For this review, take the finished solid that the model builds, in its own axes (mm). Face numbers are marked on the shaded views. A direction names the side the tool comes from. Coordinates: 2 decimals unless noted, no trailing zeros. Order: outer loops, then holes, each group sorted by start corner. A loop starts at its lowest first (then second) coordinate and runs counter-clockwise, first axis right, second up. Notation, with made-up numbers: (30, -6.5) -> (80, -6.5) arc R18 ccw to (80, 9.5) -> close; hole circle Ø3 at (54, 37.5). An arc over 180 degrees is marked (long way). Write item = value, one per line. Start each with the question number.
1) Draft analysis for pull direction Z (two halves, no side actions). For the marked faces 6, 7 and 8, state which applies: +Z half, -Z half, draft (parallel to the pull), parting line (faces both ways), or undercut.
2) Consider section A-A on x = -27. Give the boundary of the cut face in (y, z).
3) Consider section B-B on y = 17. Give the boundary of the cut face in (x, z), and give its area (3 significant figures).
4) Machinability: for the marked faces 1, 2, 3, 4 and 5, which of the approach directions +Z, -Z, +X, -X, +Y, -Y give a long, thin tool a straight path to every point of the face, cutting with its end or side? Answer none if there is none.
5) Consider section C-C on z = -17. Give the boundary of the cut face in (x, y).
6) Insertion check: pin 1 Ø5 at (x, z) = (-29, -9) entering from +Y; pin 2 Ø3 at (y, z) = (13, -1) entering from -X; pin 3 Ø3 at (x, z) = (-17.5, 9.5) entering from +Y. Each pin has a flat end and moves straight along its axis. Give the tip position at first contact, or say it passes through.
7) Consider section D-D on y = 6. Give the boundary of the cut face in (x, z).
8) Wall thickness on probe 1 along Z at (x, y) = (26, 5); probe 2 along X at (y, z) = (3, 0); probe 3 along Y at (x, z) = (-28, 7): over which ranges is each line inside the solid? List them lowest first. Write a range as [from, to].
from build123d import *

# Parameters (mm, degrees)
SALIENTE_EXTRUIR1_DEPTH = 20
CORTAR_EXTRUIR2_REACH   = 62.415
CROQUIS2_W              = 15
CROQUIS2_H              = 10


with BuildPart() as part:
    # Croquis1 → Saliente-Extruir1 (new, symmetric)
    with BuildSketch(Plane.XY):
        Polygon((-35, 0), (35, 0), (35, 10), (25, 10), (10, 45), (-10, 45), (-25, 10), (-35, 10), align=None)
    extrude(amount=SALIENTE_EXTRUIR1_DEPTH, both=True)

    # Croquis2 → Cortar-Extruir2 (cut, up to next)
    with BuildSketch(Plane.XZ, mode=Mode.PRIVATE) as cortar_extruir2_sk1:
        with Locations((27.5, 0)):
            Rectangle(CROQUIS2_W, CROQUIS2_H)
    cortar_extruir2_tool1 = extrude(cortar_extruir2_sk1.sketch, amount=-CORTAR_EXTRUIR2_REACH, mode=Mode.PRIVATE) & part.part
    # Croquis2 → Cortar-Extruir2 (cut, up to next)
    with BuildSketch(Plane.XZ, mode=Mode.PRIVATE) as cortar_extruir2_sk2:
        with Locations((-27.5, 0)):
            Rectangle(CROQUIS2_W, CROQUIS2_H)
    cortar_extruir2_tool2 = extrude(cortar_extruir2_sk2.sketch, amount=-CORTAR_EXTRUIR2_REACH, mode=Mode.PRIVATE) & part.part
    add(cortar_extruir2_tool1.solids().sort_by_distance((27.5, 0, 0))[0], mode=Mode.SUBTRACT)
    add(cortar_extruir2_tool2.solids().sort_by_distance((-27.5, 0, 0))[0], mode=Mode.SUBTRACT)


solid = part.part
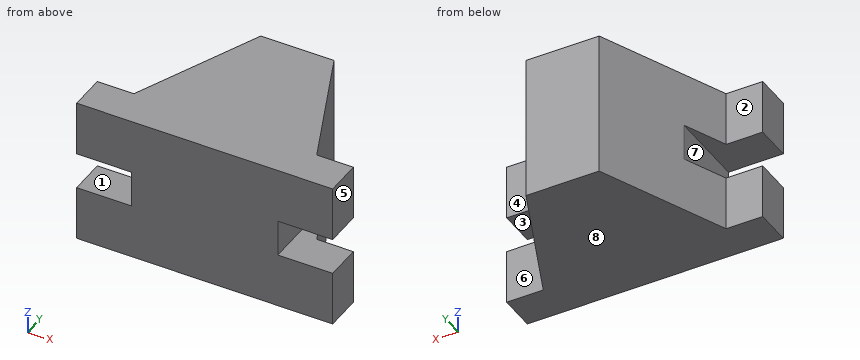
Answer sheet:
q1.face_6 = draft
q1.face_7 = undercut
q1.face_8 = -Z half
q2.outline = (0, -20) -> (10, -20) -> (10, -5) -> (0, -5) -> close; (0, 5) -> (10, 5) -> (10, 20) -> (0, 20) -> close
q3.outline = (-22, -20) -> (22, -20) -> (22, -5) -> (20, -5) -> (20, 5) -> (22, 5) -> (22, 20) -> (-22, 20) -> (-22, 5) -> (-20, 5) -> (-20, -5) -> (-22, -5) -> close
q3.area = 1,720 mm2
q4.face_1 = -X, +Y, -Y
q4.face_2 = +Z, -Z, -X, +Y
q4.face_3 = +X, +Y, -Y
q4.face_4 = +Z, -Z, +X, +Y
q4.face_5 = +Z, -Z, +X, +Y, -Y
q5.outline = (-35, 0) -> (35, 0) -> (35, 10) -> (25, 10) -> (10, 45) -> (-10, 45) -> (-25, 10) -> (-35, 10) -> close
q6.pin_1 = 10
q6.pin_2 = -20
q6.pin_3 = 31
q7.outline = (-35, -20) -> (35, -20) -> (35, -5) -> (20, -5) -> (20, 5) -> (35, 5) -> (35, 20) -> (-35, 20) -> (-35, 5) -> (-20, 5) -> (-20, -5) -> (-35, -5) -> close
q8.probe_1 = [-20, -5], [5, 20]
q8.probe_2 = [-20, 20]
q8.probe_3 = [0, 10]
